Check sheet for the drawn part. Datum: minimum x, y, z corner. Units: mm. A direction names the side the tool comes from. Give positions to 0.01 mm unless a question says otherwise; leave off trailing zeros. Order: outer loops, then holes, each group sorted by start corner. A loop starts at its lowest first (then second) coordinate and runs counter-clockwise, first axis right, second up.
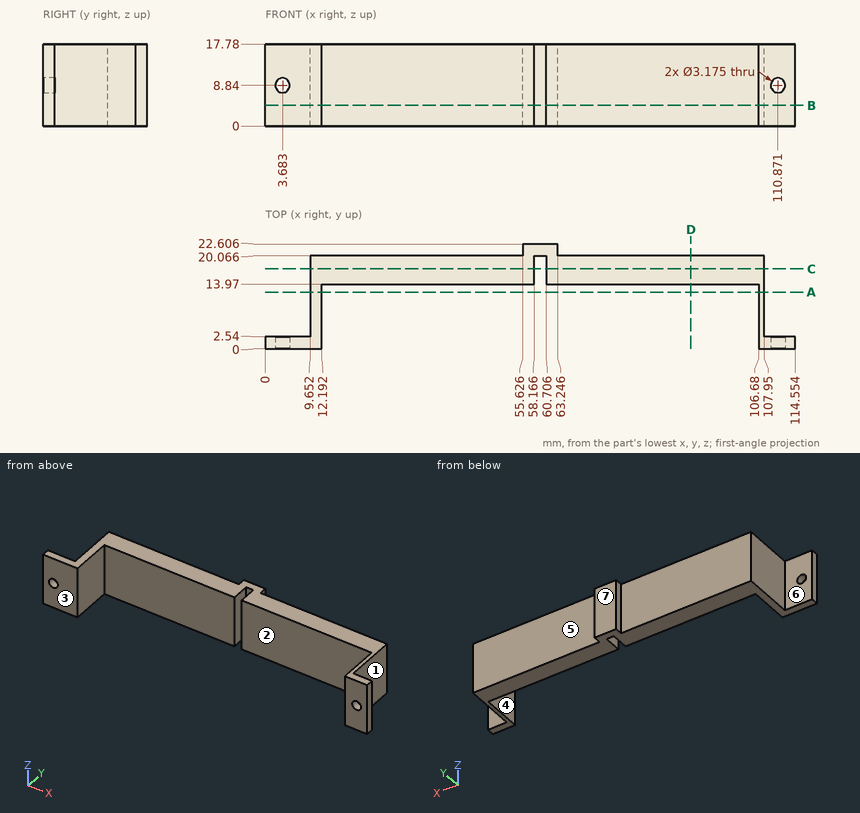
Item 1: Gauge pin test, flat ends, axial feed: pin 1 (3.5 mm diameter, centred on x = 112.5, z = 6.5, fed in from +Y); pin 2 (4 mm diameter, centred on y = 15.5, z = 3.5, fed in from +X); pin 3 (0.8 mm diameter, centred on x = 59.5, z = 7, fed in from -Y); pin 4 (3 mm diameter, centred on x = 3.68, z = 8.84, fed in from +Y). Record the tip position at first contact, or that the pin passes through.
Reported:
pin 1: stops at y = 2.54
pin 2: stops at x = 107.95
pin 3: stops at y = 20.07
pin 4: passes through
Item 2: Sectioned sample at A-A (y = 12.25). Enter the section's corners in (x, z).
Reported:
outline: (9.65, 0) - (12.19, 0) - (12.19, 17.78) - (9.65, 17.78) - close; (106.68, 0) - (107.95, 0) - (107.95, 17.78) - (106.68, 17.78) - close
Item 3: Draft check along X on the marked faces 1, 2 and 3. Enter one of: released by +X, released by -X, zero draft, split by the parting line, or undercut.
Reported:
face 1: released by +X
face 2: undercut
face 3: zero draft
Item 4: Sectioned sample at D-D (x = 92). Enter the section's corners in (y, z).
Reported:
outline: (13.97, 0) - (20.07, 0) - (20.07, 17.78) - (13.97, 17.78) - close
Item 5: Sectioned sample at C-C (y = 17.25). Enter the section's corners in (x, z), and give its area (3 significant figures).
Reported:
outline: (9.65, 0) - (58.17, 0) - (58.17, 17.78) - (9.65, 17.78) - close; (60.71, 0) - (107.95, 0) - (107.95, 17.78) - (60.71, 17.78) - close
area: 1,700 mm2
Item 6: Sectioned sample at B-B (z = 4.5). Enter the section's corners in (x, y).
Reported:
outline: (0, 0) - (12.19, 0) - (12.19, 13.97) - (58.17, 13.97) - (58.17, 20.07) - (60.71, 20.07) - (60.71, 13.97) - (106.68, 13.97) - (106.68, 0) - (114.55, 0) - (114.55, 2.54) - (107.95, 2.54) - (107.95, 20.07) - (63.25, 20.07) - (63.25, 22.61) - (55.63, 22.61) - (55.63, 20.07) - (9.65, 20.07) - (9.65, 2.54) - (0, 2.54) - close
Item 7: Scan lines: L1, parallel to X at y = 7.25, z = 13.75; L2, parallel to X at y = 15.75, z = 9.25; L3, parallel to Y at x = 53.5, z = 5. Record each from-to range of solid material in increasing order.
Reported:
L1: x = 9.65 to 12.19, 106.68 to 107.95
L2: x = 9.65 to 58.17, 60.71 to 107.95
L3: y = 13.97 to 20.07
Item 8: Set-up check for the marked faces 4, 5, 6 and 7: record each of +Z, -Z, +X, -X, +Y, -Y from which the full face is reachable in a straight line by a thin tool's end or side.
Reported:
face 4: +Z, -Z, -Y
face 5: +Z, -Z, +X, +Y
face 6: +Z, -Z, -X, +Y
face 7: +Z, -Z, +X, -X, +Y
